The model under review builds one solid part; all positions refer to its coordinate system, in mm. A direction names the side the tool comes from. Give positions to 0.01 mm unless a question says otherwise; leave off trailing zeros. Loops run counter-clockwise (first coordinate to the right, second up) from the corner with the lowest first, then second, coordinate; pieces in that order, holes last. Notation, with made-up numbers: (37.5, 23) - (70.5, 23) arc R31 cw to (70.5, 59) - close; hole circle Ø6 at (10.25, 41). An arc over 180 degrees is marked (long way). Return JSON: item names as keys, results as strings. Group by question number.
```python
from build123d import *

# Parameters (mm, degrees)
SKETCH2_R           = 10.674295377
CUT_EXTRUDE1_DEPTH  = 1.27
SKETCH3_W           = 16.858270558
SKETCH3_H           = 9.490145314
BOSS_EXTRUDE1_DEPTH = 5.08
SKETCH4_R           = 1.778
BOSS_EXTRUDE2_DEPTH = 5.08
BOSS_EXTRUDE3_START = 5.08
SKETCH5_R           = 1.778
BOSS_EXTRUDE3_DEPTH = 5.08


# Read off the part's stored shape, not the designer's step: Extrude-Thin1
with BuildPart() as part:
    # Extrude-Thin1 outline → Extrude-Thin1 (revolve)
    with BuildSketch(Plane.XZ):
        Polygon((10.16, 40.64), (0, 40.64), (0, 39.64), (7.62, 39.64), (7.62, 1), (0, 1), (0, 0), (10.16, 0), align=None)
    revolve(axis=Axis((0, 0, 0), (0, 0, 1)))

    # Sketch2 → Cut-Extrude1 (cut)
    with BuildSketch(Plane.XY.offset(40.64)):
        Circle(SKETCH2_R)
    extrude(amount=-CUT_EXTRUDE1_DEPTH, mode=Mode.SUBTRACT)

    # Sketch3 → Boss-Extrude1 (add)
    with BuildSketch(Plane(origin=(0, 0, 0), x_dir=(-1, 0, 0), z_dir=(0, 0, -1))):
        Rectangle(SKETCH3_W, SKETCH3_H)
    extrude(amount=BOSS_EXTRUDE1_DEPTH)

    # Sketch4 → Boss-Extrude2 (add)
    with BuildSketch(Plane.ZY.offset(8.429135279)):
        with Locations(Location((-2.54, 0, 0), (0, 0, 180))):
            Circle(SKETCH4_R)
    extrude(amount=BOSS_EXTRUDE2_DEPTH)

    # Sketch5 → Boss-Extrude3 (add)
    with BuildSketch(Plane(origin=(8.429135279, 0, 0), x_dir=(0, 0, -1), z_dir=(1, 0, 0)).offset(BOSS_EXTRUDE3_START)):
        with Locations((2.54, 0)):
            Circle(SKETCH5_R)
    extrude(amount=-BOSS_EXTRUDE3_DEPTH)


solid = part.part
```
1) We need section B-B, the plane x = 0. Write out the cut boundary in (y, z), plus the area to 3 significant figures.
2) We need section C-C, the plane y = 0. Write out the cut boundary in (x, z).
3) Tool access review of faces 1 (the face through (0, -4.745, -3)), 2 (the face through (0, 4.745, -3)), 3 (the face through (11, -1.08, -1.13)): name each direction out of +Z, -Z, +X, -X, +Y, -Y from which nothing blocks a thin tool from reaching the whole face with its end or side.
4) For pin 1 Ø5 at (y, z) = (-1.5, 3) entering from -X; pin 2 Ø4 at (x, z) = (3, 29.5) entering from +Y; pin 3 Ø1 at (y, z) = (2.5, 16.5) entering from -X; pin 4 Ø6 at (x, y) = (-10.5, 4) entering from +Z, all flat-tipped, find the tip position at first contact; note any pin that passes through.
5) We need section A-A, the plane z = -2.54. Write out the cut boundary in (x, y), plus the area to 3 significant figures.
6) We need section D-D, the plane z = 14.5. Write out the cut boundary in (x, y), plus the area to 3 significant figures.
7) Draft analysis for pull direction X (two halves, no side actions). For faces 4 (the face through (13.509, 0, -3)), 5 (the face through (-1.323, 10.074, 19.961)), 6 (the face through (0, 0, 1)), state which applies: +X half, -X half, draft (parallel to the pull), parting line (faces both ways), or undercut.
8) To check wall thickness, follow line 1 (Y direction, x = 0, z = 15); line 2 (Z direction, x = -6.5, y = -6); line 3 (X direction, y = 2.75, z = -0.5). State the ranges of each line that lie inside material, in increasing order.
Findings:
{
 "1": {"outline": "(-10.16, 0) - (-4.75, 0) - (-4.75, -5.08) - (4.75, -5.08) - (4.75, 0) - (10.16, 0) - (10.16, 39.37) - (7.62, 39.37) - (7.62, 1) - (-7.62, 1) - (-7.62, 39.37) - (-10.16, 39.37) - close", "area": "263 mm^2"},
 "2": {"outline": "(-13.51, -4.32) - (-8.43, -4.32) - (-8.43, -5.08) - (8.43, -5.08) - (8.43, -4.32) - (13.51, -4.32) - (13.51, -0.76) - (8.43, -0.76) - (8.43, 0) - (10.16, 0) - (10.16, 39.37) - (7.62, 39.37) - (7.62, 1) - (-7.62, 1) - (-7.62, 39.37) - (-10.16, 39.37) - (-10.16, 0) - (-8.43, 0) - (-8.43, -0.76) - (-13.51, -0.76) - close"},
 "3": {"face 1": "-Z, +X, -X, -Y", "face 2": "-Z, +X, -X, +Y", "face 3": "+X"},
 "4": {"pin 1": "stops at x = -10.16", "pin 2": "stops at y = 10.11", "pin 3": "stops at x = -9.96", "pin 4": "stops at z = 39.37"},
 "5": {"outline": "(-13.51, -1.78) - (-8.43, -1.78) - (-8.43, -4.75) - (8.43, -4.75) - (8.43, -1.78) - (13.51, -1.78) - (13.51, 1.78) - (8.43, 1.78) - (8.43, 4.75) - (-8.43, 4.75) - (-8.43, 1.78) - (-13.51, 1.78) - close", "area": "196 mm^2"},
 "6": {"outline": "circle Ø20.32 at (0, 0); hole circle Ø15.24 at (0, 0)", "area": "142 mm^2"},
 "7": {"face 4": "+X half", "face 5": "parting line", "face 6": "undercut"},
 "8": {"line 1": "y = -10.16 to -7.62, 7.62 to 10.16", "line 2": "z = 0 to 39.37", "line 3": "x = -8.43 to 8.43"}
}
